Can you work these out from the model? Positions are in its coordinate system, mm. Give positions to 0.01 mm unless a question says otherwise; leave off trailing zeros. Loops run counter-clockwise (first coordinate to the right, second up) from the corner with the lowest first, then second, coordinate; pieces in that order, holes last. Notation, with made-up numbers: (5.5, -37.5) - (20.5, -37.5) arc R22 ccw to (20.5, -13.5) - close; hole circle Ø11 at (72, -5.5). An arc over 180 degrees is marked (long way). Answer as a JSON object with one key per item and string values.
```python
from build123d import *

# Parameters (mm, degrees)
SKETCH_1_R      = 16
SKETCH_1_R_2    = 12
EXTRUDE_1_DEPTH = 14
FILLET_1_R      = 0.75


with BuildPart() as part:
    # 草图1 → 凸台-拉伸1 (new, symmetric)
    with BuildSketch(Plane(origin=(0, 0, 0), x_dir=(1, 0, 0), z_dir=(0, 1, 0))):
        with Locations(Location((0, 0, 0), (0, 0, 270))):
            Circle(SKETCH_1_R)
        with Locations(Location((0, 0, 0), (0, 0, 270))):
            Circle(SKETCH_1_R_2, mode=Mode.SUBTRACT)
    extrude(amount=EXTRUDE_1_DEPTH, both=True)

    # 圆角1
    fillet_1_edges = [part.edges().sort_by_distance(p)[0] for p in [
        (0, -14, -16),
        (0, 14, -16),
        (0, -14, -12),
        (0, 14, -12),
    ]]
    fillet(fillet_1_edges, radius=FILLET_1_R)


solid = part.part
```
1) Imagine slicing it at C-C on y = -5. Write out the boundary of the cut face in (x, z), and give its area (3 significant figures).
Check sheet entries:
{"outline": "circle Ø32 at (0, 0); hole circle Ø24 at (0, 0)", "area": "352 mm2"}
2) Imagine slicing it at A-A on x = 0. Write out the boundary of the cut face in (y, z), and give its area (3 significant figures).
Check sheet entries:
{"outline": "(-14, -15.25) arc R0.75 ccw to (-13.25, -16) - (13.25, -16) arc R0.75 ccw to (14, -15.25) - (14, -12.75) arc R0.75 ccw to (13.25, -12) - (-13.25, -12) arc R0.75 ccw to (-14, -12.75) - close; (-14, 12.75) arc R0.75 ccw to (-13.25, 12) - (13.25, 12) arc R0.75 ccw to (14, 12.75) - (14, 15.25) arc R0.75 ccw to (13.25, 16) - (-13.25, 16) arc R0.75 ccw to (-14, 15.25) - close", "area": "223 mm2"}
3) I'm going to push flat-ended pins straight in: P1, Ø12, axis at y = 8, z = -7, coming from the -X side; P2, Ø10, axis at x = -8, y = -5, coming from the +Z side; P3, Ø2, axis at x = 12, y = -6, coming from the -Z side. Where does each tip first touch, or does it pass through?
Check sheet entries:
{"P1": "x = -15.97", "P2": "z = 15.72", "P3": "z = -11.62"}
4) If we mould it in two halves opening along Z, with no side actions, what happens to faces 1 (the cylindrical face through (-15.62, 0.19, -3.47)), 2 (the cylindrical face through (3.604, -0.185, 11.446)), 3 (the flat face through (-11, -14, 7))? For each: released by +Z, released by -Z, zero draft, split by the parting line, or undercut.
Check sheet entries:
{"face 1": "split by the parting line", "face 2": "undercut", "face 3": "zero draft"}
5) Imagine slicing it at B-B on z = 0. Write out the boundary of the cut face in (x, y), and give its area (3 significant figures).
Check sheet entries:
{"outline": "(-16, -13.25) arc R0.75 ccw to (-15.25, -14) - (-12.75, -14) arc R0.75 ccw to (-12, -13.25) - (-12, 13.25) arc R0.75 ccw to (-12.75, 14) - (-15.25, 14) arc R0.75 ccw to (-16, 13.25) - close; (12, -13.25) arc R0.75 ccw to (12.75, -14) - (15.25, -14) arc R0.75 ccw to (16, -13.25) - (16, 13.25) arc R0.75 ccw to (15.25, 14) - (12.75, 14) arc R0.75 ccw to (12, 13.25) - close", "area": "223 mm2"}
6) I need wall thicknesses on L1, parallel to X at y = 4.5, z = 0; L2, parallel to Z at x = 9.5, y = 6; L3, parallel to X at y = -8, z = 3.5. Which ranges of each line are inside material? Lowest first, please.
Check sheet entries:
{"L1": "-16 to -12, 12 to 16", "L2": "-12.87 to -7.33, 7.33 to 12.87", "L3": "-15.61 to -11.48, 11.48 to 15.61"}
